Source: three-view drawing plus pictorial views. Frame: mm from the lowest corner of the part. A direction names the side the tool comes from. Give positions to 0.01 mm unless a question says otherwise; leave off trailing zeros. Write each loop counter-clockwise with the first axis right and the second up, starting at its lowest first coordinate (ties: lowest second). Pieces come first, ordered by that corner, then holes. Notation, with made-up numbers: (71.25, 83) -> (85.25, 83) arc R22 cw to (85.25, 118) -> close; hole circle Ø1 at (75.5, -23.5). An arc over 180 degrees is marked (long way). Write item = value, one per line.
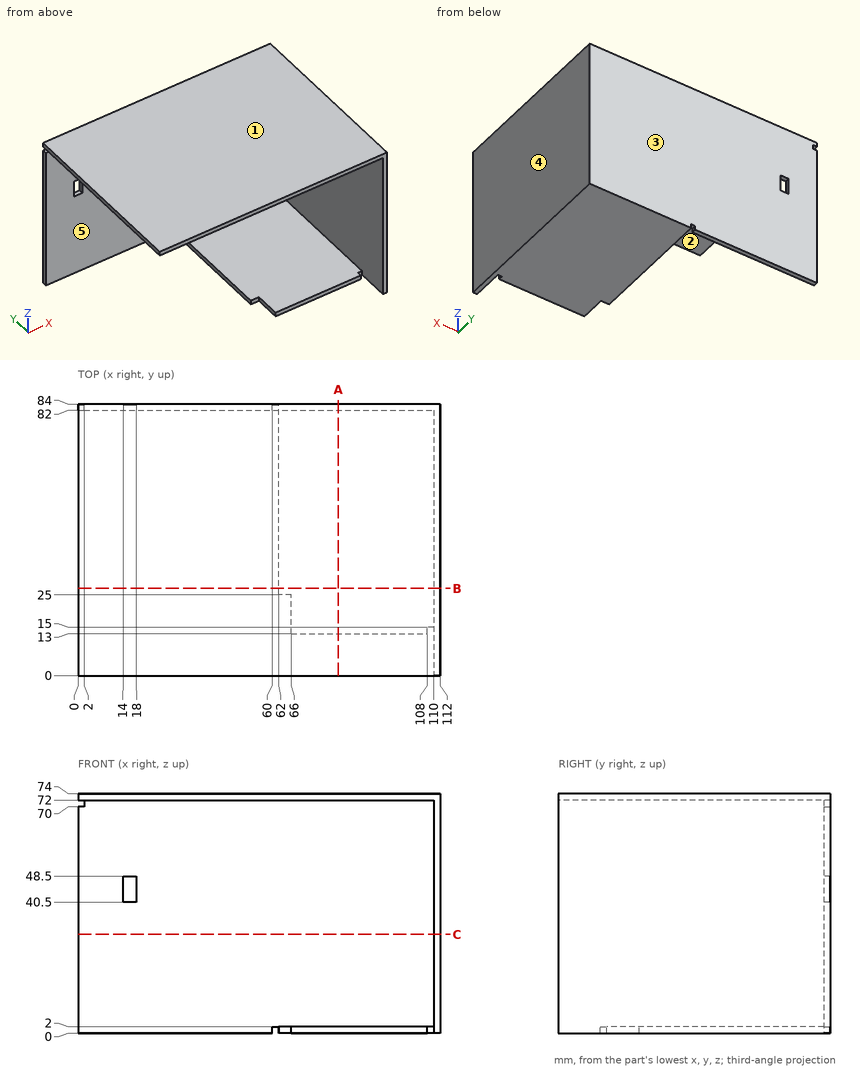
1) Material intervals for L1, parallel to Z at x = 91, y = 55; L2, parallel to Y at x = 11.5, z = 66.5; L3, parallel to Z at x = 28.5, y = 52.5, sorted ascending.
Computed:
L1 = 0 to 2, 72 to 74
L2 = 82 to 84
L3 = 72 to 74
2) Contact query for flat-ended pins moving along their axis: pin 1 (1.6 mm diameter, centred on x = 76.5, z = 0.5, fed in from -Y); pin 2 (0.6 mm diameter, centred on x = 64, z = 1.5, fed in from -Y); pin 3 (1.5 mm diameter, centred on x = 18.5, z = 41.5, fed in from -Y). Output: stop coordinate, or through.
Computed:
pin_1 = 13
pin_2 = 25
pin_3 = 82
3) Access query for the marked faces 1 and 2. Directions: +Z, -Z, +X, -X, +Y, -Y. A direction counts if a zero-diameter tool reaches every point of the face in a straight line with its end or side. Return the directions, or none.
Computed:
face_1 = +Z, +X, -X, +Y, -Y
face_2 = -X, -Y
4) Cut plane A-A (x = 80.5). Return the cut outline in (y, z).
Computed:
outline = (0, 72) -> (82, 72) -> (82, 2) -> (13, 2) -> (13, 0) -> (84, 0) -> (84, 74) -> (0, 74) -> close
5) Draft query along Y for the marked faces 3, 4 and 5. Return one class per face: pulls with the +Y half, pulls with the -Y half, needs draft (parallel to the pull), parting line crosses it, or undercut.
Computed:
face_3 = pulls with the +Y half
face_4 = needs draft
face_5 = pulls with the -Y half
6) Cut plane B-B (y = 27). Return the cut outline in (x, z).
Computed:
outline = (0, 72) -> (110, 72) -> (110, 2) -> (62, 2) -> (62, 0) -> (112, 0) -> (112, 74) -> (0, 74) -> close
7) Cut plane C-C (z = 30.5). Return the cut outline in (x, y).
Computed:
outline = (0, 82) -> (110, 82) -> (110, 0) -> (112, 0) -> (112, 84) -> (0, 84) -> close
